Autodesk Inventor part; units mm, degrees
ref_plane "YZ Plane" through (0, 0, 0) normal (1, 0, 0) x (0, 1, 0)
ref_plane "XZ Plane" through (0, 0, 0) normal (0, 1, 0) x (-1, 0, 0)
ref_plane "XY Plane" through (0, 0, 0) normal (0, 0, 1) x (1, 0, 0)
sketch "Boceto1" plane through (0, 0, 0) normal (0, 1, 0) x (-1, 0, 0)
  line L0 (-15, -2) -> (15, -2)
  line L1 (15, -2) -> (15, 2)
  line L2 (15, 2) -> (-15, 2)
  line L3 (-15, 2) -> (-15, -2)
  line L4 (-15, -2) -> (15, 2) construction
  line L5 (15, -2) -> (-15, 2) construction
  point P0 (0, 0)
  dimension "d0" = 30
  dimension "d1" = 4
extrude "Extrusión1" add sketch "Boceto1" along normal blind 60
sketch "Boceto2" plane through (-15, 0, 2) normal (0, 0, 1) x (1, 0, 0)
  line L0 (0, 60) -> (30, 60)
  line L1 (30, 0) -> (30, 60)
  line L2 (0, 60) -> (30, 60)
  line L3 (30, 60) -> (30, 56)
  line L4 (30, 56) -> (0, 56)
  line L5 (0, 56) -> (0, 60)
  point P0 (15, 0)
  dimension "d4" = 4
extrude "Extrusión2" add sketch "Boceto2" along normal blind 26
sketch "Boceto3" plane through (-15, 0, 2) normal (0, 0, 1) x (1, 0, 0)
  line L0 (0, 0) -> (30, 0)
  line L1 (0, 56) -> (30, 56)
  line L2 (0, 0) -> (3, 0)
  line L3 (3, 0) -> (3, 56)
  line L4 (3, 56) -> (0, 56)
  line L5 (0, 56) -> (0, 0)
  line L6 (30, 0) -> (27, 0)
  line L7 (27, 0) -> (27, 56)
  line L8 (27, 56) -> (30, 56)
  line L9 (30, 56) -> (30, 0)
  point P0 (15, 0)
  point P1 (3, 0)
  dimension "d7" = 3
  dimension "d8" = 3
extrude "Extrusión3" add sketch "Boceto3" along normal blind 26 contours L5 L1 L3 L0 | L7 L1 L9 L0
chamfer "Chaflán1" distance 56 distance2 26 2 edges at (-13.5, 0, 28) (13.5, 0, 28) measured on face at (-14, 38.6667, 28)
sketch "Boceto4" plane through (-12, 56, 2) normal (0, 0, 1) x (1, 0, 0)
  line L0 (27, -56) -> (-3, -56)
  line L1 (-3, -56) -> (-3, 4)
  line L2 (27, 4) -> (-3, 4)
  line L3 (27, -56) -> (27, 4)
  line L4 (-3, -56) -> (-3, 4)
  line L5 (-3, 4) -> (27, 4)
  line L6 (27, 4) -> (27, -11)
  line L7 (27, -11) -> (-3, -11)
  line L8 (-3, -11) -> (-3, 4)
  line L9 (12, -11) -> (-3, -11)
  line L10 (12, -11) -> (27, -11)
  circle A0 centre (4.5, -11) radius 1.75
  circle A1 centre (19.5, -11) radius 1.75
  line L11 (-3, -56) -> (27, -56)
  line L12 (27, -56) -> (27, -41)
  line L13 (27, -41) -> (-3, -41)
  line L14 (-3, -41) -> (-3, -56)
  line L15 (-3, -41) -> (12, -41)
  line L16 (12, -41) -> (27, -41)
  circle A2 centre (4.5, -41) radius 1.75
  circle A3 centre (19.5, -41) radius 1.75
  point P0 (12, -56)
  dimension "d14" = 30
  dimension "d15" = 15
  dimension "d16" = 3.5
  dimension "d17" = 3.5
  dimension "d18" = 30
  dimension "d19" = 15
  dimension "d20" = 15
  dimension "d21" = 15
  dimension "d22" = 3.5
  dimension "d23" = 3.5
hole "Agujero1" at (-7.5, 15, 2) at (7.5, 15, 2) at (7.5, 45, 2) at (-7.5, 45, 2) direction (0, 0, -1) diameter 3.5 end through all countersink diameter 6 countersink angle 90
properties part number "UnionBarras"
Read the model definition and answer for the solid it produces. Units are mm, in the model's axes. A direction names the side the tool comes from. Give positions to 0.01 mm unless a question says otherwise; leave off trailing zeros. Write each loop counter-clockwise with the first axis right and the second up, starting at its lowest first coordinate (ties: lowest second). Pieces come first, ordered by that corner, then holes. Notation, with made-up numbers: M 78,-13.5 L 93,-13.5 A35 ccw 93,20.5 Z; hole C 59.5,81 d2. An arc over 180 degrees is marked long. One line per item, written item: value. Start each with the question number.
(1) Find section B-B (y = 45). Determine the outline of the cut face in (x, z).
(2) Find section A-A (x = -7.5). Determine the outline of the cut face in (y, z), plus the area to 3 significant figures.
(3) Flat-ended cylindrical pins translate along their axes: pin 1 Ø12 at (x, z) = (-3, 18) entering from -Y; pin 2 Ø3 at (x, y) = (-7.5, 15) entering from +Z; pin 3 Ø12 at (x, y) = (-1.5, 30) entering from +Z; pin 4 Ø4 at (x, y) = (7.5, 45) entering from +Z. Find the tip coordinate at first contact, or state that the pin passes through.
(4) Find the intervals of material crossed by line 1 (Y direction, x = 7.5, z = -0.5); line 2 (X direction, y = 15, z = -0.9); line 3 (X direction, y = 14, z = 8), in increasing order.
(5) Find section C-C (z = 26). Determine the outline of the cut face in (x, y).
(6) A tool of negligible diameter and unlimited length cuts with its end or side. For faces 1 (the cylindrical face through (8.17, 43.383, -0.644)), 2 (the flat face through (12, 40, 9)), from which of +Z, -Z, +X, -X, +Y, -Y can it reach the whole face along a straight path? Write none if from no direction.
(7) Find section D-D (x = -3). Determine the outline of the cut face in (y, z), plus the area to 3 significant figures.
Results below:
1. outline: M -15,-2 L -9.25,-2 L -9.25,0.75 L -10.5,2 L -12,2 L -12,22.89 L -15,22.89 Z; M -5.75,-2 L 5.75,-2 L 5.75,0.75 L 4.5,2 L -4.5,2 L -5.75,0.75 Z; M 9.25,-2 L 15,-2 L 15,22.89 L 12,22.89 L 12,2 L 10.5,2 L 9.25,0.75 Z
2. outline: M 0,-2 L 13.25,-2 L 13.25,0.75 L 12,2 L 0,2 Z; M 16.75,-2 L 43.25,-2 L 43.25,0.75 L 42,2 L 18,2 L 16.75,0.75 Z; M 46.75,-2 L 60,-2 L 60,28 L 56,28 L 56,2 L 48,2 L 46.75,0.75 Z
2. area: 313 mm^2
3. pin 1: stops at y = 56
3. pin 2: passes through
3. pin 3: stops at z = 2
3. pin 4: stops at z = 1
4. line 1: y = 0 to 13.25, 16.75 to 43.25, 46.75 to 60
4. line 2: x = -15 to -9.25, -5.75 to 5.75, 9.25 to 15
4. line 3: x = -15 to -12, 12 to 15
5. outline: M -15,51.69 L -12,51.69 L -12,56 L 12,56 L 12,51.69 L 15,51.69 L 15,60 L -15,60 Z
6. face 1: +Z, -Z
6. face 2: +Z, -Y
7. outline: M 0,-2 L 60,-2 L 60,28 L 56,28 L 56,2 L 0,2 Z
7. area: 344 mm^2
